Part model, mm, in its own coordinate system. Face numbers are marked on the shaded views. Coordinates: 2 decimals unless noted, no trailing zeros. Loops run counter-clockwise (first coordinate to the right, second up) from the corner with the lowest first, then second, coordinate; pieces in that order, holes last. Notation, with made-up numbers: M 9,32 L 28,32 A11 ccw 28,45 Z; hole C 42,-8 d4. An arc over 180 degrees is marked long. Answer as a JSON object with one key per item and string values. Group by question number.
1. Saw through at A-A on y = 0. Write the cut outline in (x, z).
2. Mould opens along X. For the marked faces 1, 2, 3 and 4 say: released by +X, released by -X, zero draft, split by the parting line, or undercut.
3. Saw through at D-D on x = 6.25. Write the cut outline in (y, z).
4. Drop flat-ended pins along their axis: pin 1 Ø3 at (x, y) = (2.5, 5.5) entering from -Z; pin 2 Ø5 at (x, y) = (-0.5, 2) entering from +Z; pin 3 Ø9 at (x, y) = (0, 0) entering from +Z; pin 4 Ø8 at (y, z) = (5.5, 7.5) entering from +X. Give the stop position or say it passes through.
5. Drill centre lines: L1, parallel to Y at x = 0, z = 5; L2, parallel to X at y = -1.5, z = 8.75; L3, parallel to X at y = -1.25, z = 14. Where is each one in solid material? Low to high.
6. Saw through at C-C on z = 15. Write the cut outline in (x, y).
from build123d import *

# Parameters (mm, degrees)
SKETCH_1_R        = 8
EXTRUDE_1_DEPTH   = 20
HOLE_WIZARD_M81_D = 6.8
CHAMFER_1_SIZE    = 2


with BuildPart() as part:
    # Эскиз1 → Бобышка-Вытянуть1 (new body)
    with BuildSketch(Plane.XY):
        Circle(SKETCH_1_R)
    extrude(amount=EXTRUDE_1_DEPTH)

    # Отверстие обработанное метчиком M81 (through all)
    with Locations(Plane.XY.offset(20)):
        with Locations((0, 0)):
            Hole(HOLE_WIZARD_M81_D / 2)

    # Фаска1
    chamfer_1_edges = [part.edges().sort_by_distance(p)[0] for p in [
        (3.4, 0, 20),
    ]]
    chamfer(chamfer_1_edges, length=CHAMFER_1_SIZE)


solid = part.part
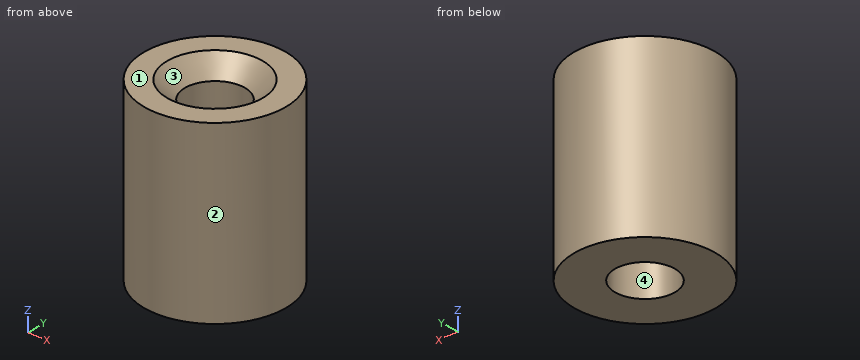
Outcome:
{
 "1": {"outline": "M -8,0 L -3.4,0 L -3.4,18 L -5.4,20 L -8,20 Z; M 3.4,0 L 8,0 L 8,20 L 5.4,20 L 3.4,18 Z"},
 "2": {"face 1": "zero draft", "face 2": "split by the parting line", "face 3": "undercut", "face 4": "undercut"},
 "3": {"outline": "M -4.99,0 L 4.99,0 L 4.99,20 L -4.99,20 Z"},
 "4": {"pin 1": "stops at z = 0", "pin 2": "stops at z = 19.16", "pin 3": "stops at z = 19.1", "pin 4": "stops at x = 7.86"},
 "5": {"L1": "y = -8 to -3.4, 3.4 to 8", "L2": "x = -7.86 to -3.05, 3.05 to 7.86", "L3": "x = -7.9 to -3.16, 3.16 to 7.9"},
 "6": {"outline": "C 0,0 d16; hole C 0,0 d6.8"}
}
